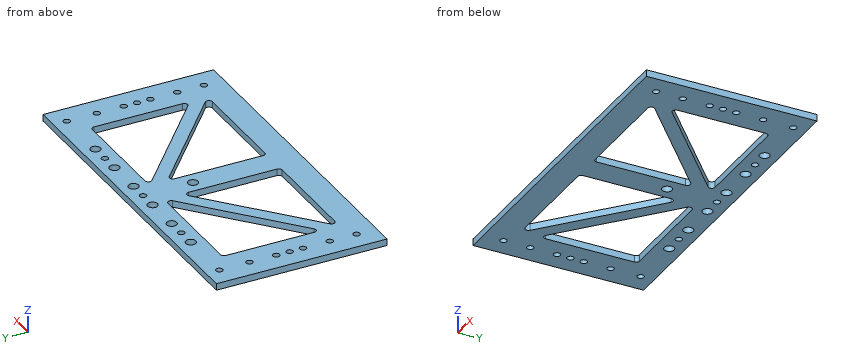
from build123d import *

# Parameters (mm, degrees)
SKETCH1_W                   = 635
SKETCH1_H                   = 323.85
BOSS_EXTRUDE1_DEPTH         = 12.7
F_3_4_0_75_DIAMETER_HOLE1_D = 19.05
F_1_2_0_5_DIAMETER_HOLE1_D  = 12.7
LPATTERN1_COUNT             = 2
LPATTERN1_PITCH             = 558.8
LPATTERN1_COUNT_DIR2        = 5
LPATTERN1_PITCH_DIR2        = 50.8
HOLE1_OUTLINE_R             = 9.525
HOLE1_DEPTH                 = 12.7
LPATTERN2_COUNT             = 6
LPATTERN2_PITCH             = 69.85
HOLE2_OUTLINE_R             = 6.35
HOLE2_DEPTH                 = 12.7
LPATTERN3_COUNT             = 5
LPATTERN3_PITCH             = 139.7
CUT_EXTRUDE1_DEPTH          = 713.927143893
FILLET1_R                   = 6.35
F_1_2_0_5_DIAMETER_HOLE2_D  = 12.7


# Read off the part's stored shape, not the designer's step: Hole1, Hole2
with BuildPart() as part:
    # Sketch1 → Boss-Extrude1 (new body)
    with BuildSketch(Plane.XY):
        with Locations((317.5, 161.925)):
            Rectangle(SKETCH1_W, SKETCH1_H)
    extrude(amount=BOSS_EXTRUDE1_DEPTH)

    # 3/4 (0.75) Diameter Hole1 (through all)
    with Locations(Plane.XY.offset(12.7)):
        with Locations((317.5, 203.85)):
            Hole(F_3_4_0_75_DIAMETER_HOLE1_D / 2)

    # 1/2 (0.5) Diameter Hole1 (through all)
    with Locations(Plane.XY.offset(12.7)):
        with Locations((38.1, 38.1)):
            f_1_2_0_5_diameter_hole1 = Hole(F_1_2_0_5_DIAMETER_HOLE1_D / 2)

    # LPattern1: 1_2 _0.5_ Diameter Hole1 2 × 5
    with Locations(*[(i * LPATTERN1_PITCH, j * LPATTERN1_PITCH_DIR2, 0) for i in range(LPATTERN1_COUNT) for j in range(LPATTERN1_COUNT_DIR2) if (i, j) != (0, 0)]):
        add(f_1_2_0_5_diameter_hole1, mode=Mode.SUBTRACT)

    # Hole1 outline → Hole1 (cut)
    with BuildSketch(Plane.XY):
        with Locations((142.875, 298.45)):
            Circle(HOLE1_OUTLINE_R)
    hole1 = extrude(amount=HOLE1_DEPTH, mode=Mode.SUBTRACT)

    # LPattern2: Hole1 ×6
    with Locations(*[(i * LPATTERN2_PITCH, 0, 0) for i in range(1, LPATTERN2_COUNT)]):
        add(hole1, mode=Mode.SUBTRACT)

    # Hole2 outline → Hole2 (cut)
    with BuildSketch(Plane.XY):
        with Locations((38.1, 298.45)):
            Circle(HOLE2_OUTLINE_R)
    hole2 = extrude(amount=HOLE2_DEPTH, mode=Mode.SUBTRACT)

    # LPattern3: Hole2 ×5
    with Locations(*[(i * LPATTERN3_PITCH, 0, 0) for i in range(1, LPATTERN3_COUNT)]):
        add(hole2, mode=Mode.SUBTRACT)

    # Sketch9 → Cut-Extrude1 (cut, through all)
    with BuildSketch(Plane.XY.offset(12.7)):
        Polygon((76.2, 273.05), (292.1, 273.05), (76.2, 84.521018444), align=None)
        Polygon((76.2, 50.8), (292.1, 239.328981556), (292.1, 50.8), align=None)
        Polygon((342.9, 273.05), (558.8, 273.05), (558.8, 84.521018444), align=None)
        Polygon((342.9, 239.328981556), (342.9, 50.8), (558.8, 50.8), align=None)
    extrude(amount=-CUT_EXTRUDE1_DEPTH, mode=Mode.SUBTRACT)

    # Fillet1
    fillet1_edges = [part.edges().sort_by_distance(p)[0] for p in [
        (292.1, 50.8, 6.35),
        (76.2, 50.8, 6.35),
        (292.1, 239.328981556, 6.35),
        (558.8, 84.521018444, 6.35),
        (342.9, 273.05, 6.35),
        (558.8, 273.05, 6.35),
        (342.9, 239.328981556, 6.35),
        (558.8, 50.8, 6.35),
        (342.9, 50.8, 6.35),
        (76.2, 84.521018444, 6.35),
        (76.2, 273.05, 6.35),
        (292.1, 273.05, 6.35),
    ]]
    fillet(fillet1_edges, radius=FILLET1_R)

    # 1/2 (0.5) Diameter Hole2 (through all)
    with Locations(Plane.XY.offset(12.7)):
        with Locations((38.1, 165.1), (596.9, 165.1)):
            Hole(F_1_2_0_5_DIAMETER_HOLE2_D / 2)


solid = part.part
Source: CAD feature listing. Evaluate the final solid. Frame: model axes, mm. Round coordinates to 2 decimals unless told otherwise and drop trailing zeros. Loops run counter-clockwise (first coordinate to the right, second up) from the corner with the lowest first, then second, coordinate; pieces in that order, holes last.
Q1. Section D-D, the plane x = 369. Return loops of the section in (y, z).
Q2. First-contact query: P1, Ø16.5, axis at x = 38.1, y = 88.9, coming from the +Z side; P2, Ø11.5, axis at x = 38.1, y = 190.5, coming from the -Z side. Flat tips, straight axial feed; report the tip coordinate or a pass-through.
Q3. Ray query, line 1 (X direction, y = 104.5, z = 10); line 2 (X direction, y = 176, z = 3.75); line 3 (X direction, y = 42, z = 6.5). Return the intervals inside material, ascending.
Q4. Section A-A, the plane x = 38.1. State how many separate pieces and enclosed holes the cut face has, plus the area to 3 significant figures.
Q5. Section B-B, the plane y = 165.1. Return loops of the section in (x, z), plus the area to 3 significant figures.
Q6. Section C-C, the plane y = 38.1. Return loops of the section in (x, z), plus the area to 3 significant figures.
Solutions:
1. outline: (0, 0) - (50.8, 0) - (50.8, 12.7) - (0, 12.7) - close; (216.54, 0) - (250.26, 0) - (250.26, 12.7) - (216.54, 12.7) - close; (273.05, 0) - (323.85, 0) - (323.85, 12.7) - (273.05, 12.7) - close
2. P1: stops at z = 12.7
2. P2: passes through
3. line 1: x = 0 to 76.2, 99.08 to 137.7, 292.1 to 342.9, 497.3 to 535.92, 558.8 to 635
3. line 2: x = 0 to 76.2, 180.96 to 219.58, 292.1 to 342.9, 415.42 to 454.04, 558.8 to 635
3. line 3: x = 0 to 33.09, 43.11 to 591.89, 601.91 to 635
4. separate pieces: 8
4. enclosed holes: 0
4. area: 2,980 mm2
5. outline: (0, 0) - (31.75, 0) - (31.75, 12.7) - (0, 12.7) - close; (44.45, 0) - (76.2, 0) - (76.2, 12.7) - (44.45, 12.7) - close; (168.48, 0) - (207.09, 0) - (207.09, 12.7) - (168.48, 12.7) - close; (292.1, 0) - (342.9, 0) - (342.9, 12.7) - (292.1, 12.7) - close; (427.91, 0) - (466.52, 0) - (466.52, 12.7) - (427.91, 12.7) - close; (558.8, 0) - (590.55, 0) - (590.55, 12.7) - (558.8, 12.7) - close; (603.25, 0) - (635, 0) - (635, 12.7) - (603.25, 12.7) - close
5. area: 3,240 mm2
6. outline: (0, 0) - (31.75, 0) - (31.75, 12.7) - (0, 12.7) - close; (44.45, 0) - (590.55, 0) - (590.55, 12.7) - (44.45, 12.7) - close; (603.25, 0) - (635, 0) - (635, 12.7) - (603.25, 12.7) - close
6. area: 7,740 mm2
